from build123d import *

# Parameters (mm, degrees)
F1_DEPTH = 2.9718


with BuildPart() as f1:
    # F0 (on Right) → F1 (new body)
    with BuildSketch(Plane.YZ):
        Polygon((0, 10.795), (0, 0), (18.8468, 0), (18.8468, 6.985), (16.9418, 6.985), (16.9418, 9.525), (18.8468, 9.525), (18.8468, 13.97), (22.6568, 13.97), (22.6568, 9.525), (24.5618, 9.525), (24.5618, 6.985), (22.6568, 6.985), (22.6568, 0), (80.6196, 0), (80.6196, 6.985), (78.7146, 6.985), (78.7146, 9.525), (80.6196, 9.525), (80.6196, 13.97), (84.4296, 13.97), (84.4296, 9.525), (86.3346, 9.525), (86.3346, 6.985), (84.4296, 6.985), (84.4296, 0), (103.2764, 0), (103.2764, 10.795), (96.2914, 10.795), (96.2914, 8.89), (93.7514, 8.89), (93.7514, 10.795), (89.3064, 10.795), (89.3064, 14.605), (93.7514, 14.605), (93.7514, 16.51), (96.2914, 16.51), (96.2914, 14.605), (103.2764, 14.605), (103.2764, 49.53), (96.2914, 49.53), (96.2914, 47.625), (93.7514, 47.625), (93.7514, 49.53), (89.3064, 49.53), (89.3064, 53.34), (93.7514, 53.34), (93.7514, 55.245), (96.2914, 55.245), (96.2914, 53.34), (103.2764, 53.34), (103.2764, 60.96), (0, 60.96), (0, 53.34), (6.985, 53.34), (6.985, 55.245), (9.525, 55.245), (9.525, 53.34), (13.97, 53.34), (13.97, 49.53), (9.525, 49.53), (9.525, 47.625), (6.985, 47.625), (6.985, 49.53), (0, 49.53), (0, 14.605), (6.985, 14.605), (6.985, 16.51), (9.525, 16.51), (9.525, 14.605), (13.97, 14.605), (13.97, 10.795), (9.525, 10.795), (9.525, 8.89), (6.985, 8.89), (6.985, 10.795), align=None)
    extrude(amount=F1_DEPTH)


solid = f1.part
Can you work these out from the model? Positions are in its coordinate system, mm. A direction names the side the tool comes from. Round coordinates to 2 decimals unless told otherwise and drop trailing zeros. Order: outer loops, then holes, each group sorted by start corner. A loop starts at its lowest first (then second) coordinate and runs counter-clockwise, first axis right, second up. Notation, with made-up numbers: (-6, 89.25) - (50, 89.25) arc R16 cw to (50, 117.25) - close; hole circle Ø5 at (88, 69.25). An arc over 180 degrees is marked (long way). Answer in a Markdown table with one row per item.
(1) If we mould it in two halves opening along Z, with no side actions, what happens to faces 1 (the face through (1, 94, 0)), 2 (the face through (1, 93.751, 54)), 3 (the face through (0, 51, 31))? For each: released by +Z, released by -Z, zero draft, split by the parting line, or undercut.
From the geometry:
| item | result |
|---|---|
| face 1 | released by -Z |
| face 2 | undercut |
| face 3 | zero draft |
(2) Which directions (+Z, -Z, +X, -X, +Y, -Y) give clear straight access to the entire face, cutting with the end or side of a thin tool? Please do faces 4 (the face through (1, 4, 49.53)), 5 (the face through (1, 100, 14.605)), 6 (the face through (1, 6.985, 16)).
From the geometry:
| item | result |
|---|---|
| face 4 | +X, -X, -Y |
| face 5 | +X, -X, +Y |
| face 6 | +X, -X |
(3) Suppose I cut it at B-B, the plane z = 51. Please give me the cut outline in (x, y), plus the area to 3 significant figures.
From the geometry:
| item | result |
|---|---|
| outline | (0, 13.97) - (2.97, 13.97) - (2.97, 89.31) - (0, 89.31) - close |
| area | 224 mm2 |
(4) For P1, Ø0.9, axis at x = 1, z = 12.5, coming from the -Y side; P2, Ø0.9, axis at x = 2, y = 82.5, coming from the -Z side; P3, Ø0.8, axis at x = 1, z = 8.5, coming from the -Y side, each with a flat end and sliding along its axis, tell me the tip position at first contact or that it passes through.
From the geometry:
| item | result |
|---|---|
| P1 | stops at y = 13.97 |
| P2 | stops at z = 13.97 |
| P3 | stops at y = 0 |
(5) Please list where these lines run through material, in increasing order: L1, parallel to Z at x = 0.75, y = 97 (3 decimals); L2, parallel to Z at x = 2.8, y = 8.5 (3 decimals); L3, parallel to Y at x = 2.8, z = 48 (3 decimals). Write a range as from..to.
From the geometry:
| item | result |
|---|---|
| L1 | z = 0..10.795, 14.605..49.53, 53.34..60.96 |
| L2 | z = 0..8.89, 16.51..47.625, 55.245..60.96 |
| L3 | y = 0..6.985, 9.525..93.751, 96.291..103.276 |
(6) Suppose I cut it at A-A, the plane y = 91.5. Please give me the cut outline in (x, z) (3 decimals), plus the area to 3 significant figures.
From the geometry:
| item | result |
|---|---|
| outline | (0, 0) - (2.972, 0) - (2.972, 10.795) - (0, 10.795) - close; (0, 14.605) - (2.972, 14.605) - (2.972, 49.53) - (0, 49.53) - close; (0, 53.34) - (2.972, 53.34) - (2.972, 60.96) - (0, 60.96) - close |
| area | 159 mm2 |
